Input: dimensioned drawing with shaded views. Units: mm. Origin: part minimum x, y, z. A direction names the side the tool comes from. Round coordinates to 2 decimals unless told otherwise and drop trailing zeros. Loops run counter-clockwise (first coordinate to the right, second up) from the corner with the lowest first, then second, coordinate; pieces in that order, holes last.
Item 1: Access query for the marked faces 1, 2, 3 and 4. Directions: +Z, -Z, +X, -X, +Y, -Y. A direction counts if a zero-diameter tool reaches every point of the face in a straight line with its end or side. Return the directions, or none.
Item 2: First-contact query: P1, Ø0.5, axis at y = 0.5, z = 2.5, coming from the +X side; P2, Ø0.7, axis at x = 3, y = 1, coming from the -Z side; P3, Ø1.1, axis at x = 4.5, y = 1.5, coming from the +Z side. Flat tips, straight axial feed; report the tip coordinate or a pass-through.
Item 3: Section query A-A on y = 2.35. Return loops of the section in (x, z).
Item 4: Ray query, L1, parallel to X at y = 1.65, z = 1.9; L2, parallel to Z at x = 4, y = 1.6; L3, parallel to Y at x = 7, z = 1.35. Return the intervals inside material, ascending.
Item 5: Section query B-B on x = 5.75. Return loops of the section in (y, z), then the cut area to 3 significant figures.
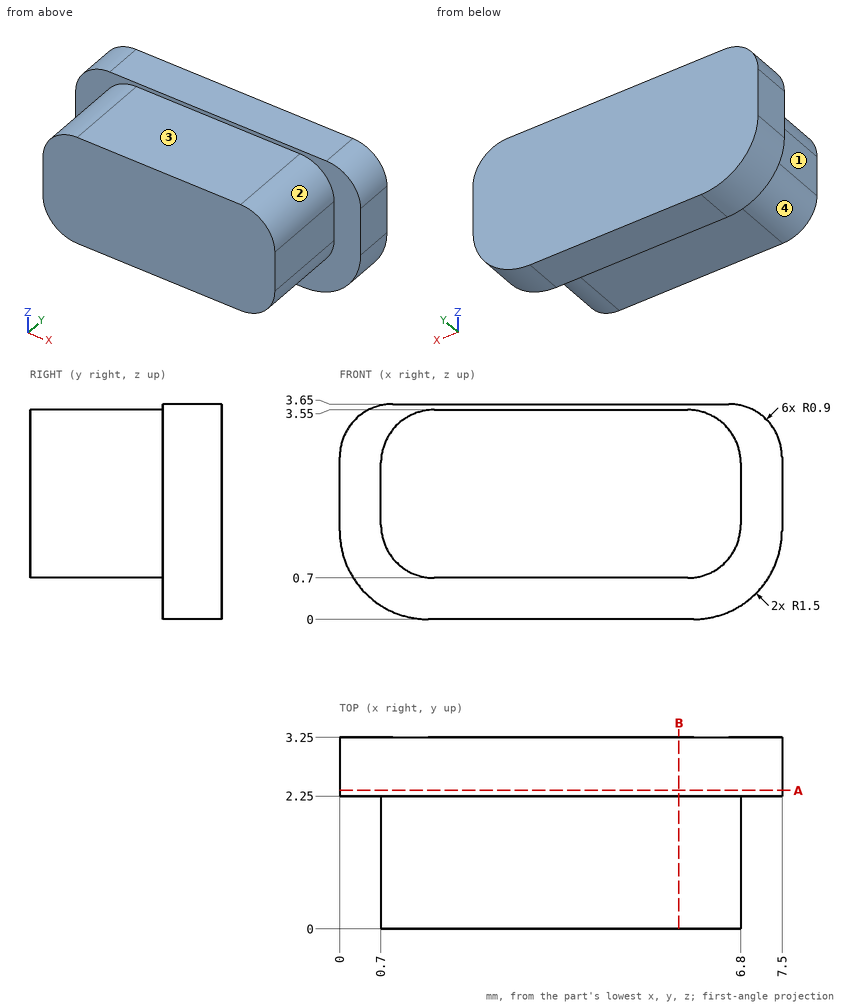
Data:
1. face 1: +Z, -Z, -X, -Y
1. face 2: +Z, +X, -Y
1. face 3: +Z, +X, -X, -Y
1. face 4: -Z, -X, -Y
2. P1: stops at x = 6.8
2. P2: stops at z = 0.7
2. P3: stops at z = 3.55
3. outline: (0, 1.5) arc R1.5 ccw to (1.5, 0) - (6, 0) arc R1.5 ccw to (7.5, 1.5) - (7.5, 2.75) arc R0.9 ccw to (6.6, 3.65) - (0.9, 3.65) arc R0.9 ccw to (0, 2.75) - close
4. L1: x = 0.7 to 6.8
4. L2: z = 0.7 to 3.55
4. L3: y = 2.25 to 3.25
5. outline: (0, 0.7) - (2.25, 0.7) - (2.25, 0) - (3.25, 0) - (3.25, 3.65) - (2.25, 3.65) - (2.25, 3.55) - (0, 3.55) - close
5. area: 10.1 mm2
